```python
from build123d import *

# Parameters (mm, degrees)
SKETCH1_R           = 0.375
SKETCH1_R_2         = 3.5
BOSS_EXTRUDE1_DEPTH = 0.1


with BuildPart() as part:
    # Sketch1 → Boss-Extrude1 (new body, symmetric)
    with BuildSketch(Plane.XY):
        with BuildLine():
            Line((-0.636628274, -7.407290054), (3.704019046, 3.239952681))
            ThreePointArc((3.704019046, 3.239952681), (3.507926477, 6.672095687), (0.720779018, 8.68452381))
            ThreePointArc((0.720779018, 8.68452381), (0, 11.5), (-0.720779018, 8.68452381))
            ThreePointArc((-0.720779018, 8.68452381), (-3.983597321, 4.388126568), (0, 0.75))
            Line((0, 0.75), (2.148965927, 0.75))
            Line((2.148965927, 0.75), (-1.099630654, -7.218534139))
            ThreePointArc((-1.099630654, -7.218534139), (-1.165325631, -7.4384166), (-1.1875, -7.666829437))
            Line((-1.1875, -7.666829437), (-1.1875, -9.083570106))
            ThreePointArc((-1.1875, -9.083570106), (0.960377242, -11.152248043), (-0.6875, -8.666829437))
            Line((-0.6875, -8.666829437), (-0.6875, -7.666829437))
            ThreePointArc((-0.6875, -7.666829437), (-0.674662207, -7.534590426), (-0.636628274, -7.407290054))
        make_face()
        with Locations((0, -10)):
            Circle(SKETCH1_R, mode=Mode.SUBTRACT)
        with Locations((0, 10)):
            Circle(SKETCH1_R, mode=Mode.SUBTRACT)
        with Locations((0, 4.75)):
            Circle(SKETCH1_R_2, mode=Mode.SUBTRACT)
    extrude(amount=BOSS_EXTRUDE1_DEPTH, both=True)


solid = part.part
```
The listing builds one solid part. Answer for the finished solid, in the listing's coordinates (mm). Round coordinates to 2 decimals unless told otherwise and drop trailing zeros. Loops run counter-clockwise (first coordinate to the right, second up) from the corner with the lowest first, then second, coordinate; pieces in that order, holes last.
Q1. Find the intervals of material crossed by line 1 (Y direction, x = 0, z = 0.05) (3 decimals); line 2 (Y direction, x = 2.25, z = 0.05); line 3 (Y direction, x = -1.75, z = 0), in increasing order.
Q2. Section B-B, the plane x = -2.75 is taken. Determine the outline of the cut face in (y, z), then the cut area to 3 significant figures.
Q3. Section A-A, the plane y = 4.75 is taken. Determine the outline of the cut face in (x, z), then the cut area to 3 significant figures.
Q4. Section C-C, the plane x = 1.25 is taken. Determine the outline of the cut face in (y, z), then the cut area to 3 significant figures.
Q5. Section D-D, the plane y = 0.25 is taken. Determine the outline of the cut face in (x, z).
Completed:
1. line 1: y = -11.5 to -10.375, -9.625 to -8.5, -5.846 to -4.521, 0.75 to 1.25, 8.25 to 9.625, 10.375 to 11.5
1. line 2: y = -0.33 to 2.07, 7.43 to 8.06
1. line 3: y = 1.15 to 1.72, 7.78 to 8.35
2. outline: (1.85, -0.1) - (2.58, -0.1) - (2.58, 0.1) - (1.85, 0.1) - close; (6.92, -0.1) - (7.65, -0.1) - (7.65, 0.1) - (6.92, 0.1) - close
2. area: 0.296 mm2
3. outline: (-4, -0.1) - (-3.5, -0.1) - (-3.5, 0.1) - (-4, 0.1) - close; (3.5, -0.1) - (4, -0.1) - (4, 0.1) - (3.5, 0.1) - close
3. area: 0.200 mm2
4. outline: (-10.83, -0.1) - (-9.17, -0.1) - (-9.17, 0.1) - (-10.83, 0.1) - close; (-2.78, -0.1) - (-1.46, -0.1) - (-1.46, 0.1) - (-2.78, 0.1) - close; (0.75, -0.1) - (1.48, -0.1) - (1.48, 0.1) - (0.75, 0.1) - close; (8.02, -0.1) - (8.55, -0.1) - (8.55, 0.1) - (8.02, 0.1) - close; (9.17, -0.1) - (10.83, -0.1) - (10.83, 0.1) - (9.17, 0.1) - close
4. area: 1.18 mm2
5. outline: (1.95, -0.1) - (2.49, -0.1) - (2.49, 0.1) - (1.95, 0.1) - close
